Read the model definition and answer for the solid it produces. Units are mm, in the model's axes. A direction names the side the tool comes from. Round coordinates to 2 decimals unless told otherwise and drop trailing zeros. Order: outer loops, then holes, each group sorted by start corner. A loop starts at its lowest first (then second) coordinate and runs counter-clockwise, first axis right, second up. Notation, with made-up numbers: M 51.25,-30.5 L 81.25,-30.5 A18 cw 81.25,-9.5 Z; hole C -17,-3 d7. An arc over 180 degrees is marked long. Answer as CSV lines item,"result".
```python
from build123d import *

# Parameters (mm, degrees)
BOSS_EXTRUDE1_DEPTH = 9
CUT_EXTRUDE1_DEPTH  = 1.5


with BuildPart() as part:
    # Sketch1 → Boss-Extrude1 (new, symmetric)
    with BuildSketch(Plane.XY):
        with BuildLine():
            Line((-0.064848747, 6.937253933), (-8.564848747, 6.937253933))
            Line((-8.564848747, 6.937253933), (-8.564848747, 7.937253933))
            Line((-8.564848747, 7.937253933), (0, 7.937253933))
            ThreePointArc((0, 7.937253933), (5, 5.291502622), (7, 0))
            ThreePointArc((7, 0), (6.838022738, -1.497145631), (6.359587132, -2.925004532))
            Line((6.359587132, -2.925004532), (5.451074684, -2.507146742))
            ThreePointArc((5.451074684, -2.507146742), (5.861162347, -1.283267683), (6, 0))
            ThreePointArc((6, 0), (4.270012276, 4.607273664), (-0.064848747, 6.937253933))
        make_face()
    extrude(amount=BOSS_EXTRUDE1_DEPTH, both=True)

    # Sketch2 → Cut-Extrude1 (cut)
    with BuildSketch(Plane.XY.offset(9)):
        with BuildLine():
            Line((5.451074684, -2.507146742), (6.359587132, -2.925004532))
            ThreePointArc((6.359587132, -2.925004532), (6.838022738, -1.497145631), (7, 0))
            ThreePointArc((7, 0), (5.923664522, 4.007850993), (2.984282604, 6.937253933))
            Line((2.984282604, 6.937253933), (-0.064848747, 6.937253933))
            ThreePointArc((-0.064848747, 6.937253933), (4.270012276, 4.607273664), (6, 0))
            ThreePointArc((6, 0), (5.861162347, -1.283267683), (5.451074684, -2.507146742))
        make_face()
    cut_extrude1 = extrude(amount=-CUT_EXTRUDE1_DEPTH, mode=Mode.SUBTRACT)

    # Mirror1: Cut-Extrude1 across plane
    add(cut_extrude1.mirror(Plane.XY), mode=Mode.SUBTRACT)


solid = part.part
```
Item 1: A tool of negligible diameter and unlimited length cuts with its end or side. For faces 4 (the face through (-2.7, 7.4, -9)), 5 (the face through (4.32, 4.55, 0.11)), 6 (the face through (6, 3, -7.5)), 7 (the face through (6, 3, 7.5)), from which of +Z, -Z, +X, -X, +Y, -Y can it reach the whole face along a straight path? Write none if from no direction.
Ans:
face 4,"-Z, +X, -X, +Y, -Y"
face 5,"+Z, -Z, -X"
face 6,"-Z, +X, -X, -Y"
face 7,"+Z, +X, -X, -Y"
Item 2: Find the intervals of material crossed by probe 1 along Y at (x, z) = (-6.75, -7.5); probe 2 along X at (y, z) = (3.75, -5); probe 3 along X at (y, z) = (5.5, 2.5), in increasing order. Write a range as [from, to].
Ans:
probe 1,"[6.94, 7.94]"
probe 2,"[4.91, 6.07]"
probe 3,"[3.33, 4.81]"
Item 3: Determine the mould class of faces 1 (the face through (4.9, 5.4, 0.1)), 2 (the face through (-4, 6.937, 0)), 3 (the face through (5.857, -1.301, 0.105)) for opening direction Y: +Y half, -Y half, draft (parallel to the pull), parting line (faces both ways), or undercut.
Ans:
face 1,"+Y half"
face 2,"-Y half"
face 3,"undercut"
Item 4: A cutting plane is placed at B-B, the plane x = 1.25. Determine the outline of the cut face in (y, z).
Ans:
outline,"M 6.63,-7.5 L 6.94,-7.5 L 6.94,-9 L 7.68,-9 L 7.68,9 L 6.94,9 L 6.94,7.5 L 6.63,7.5 Z"
Item 5: A cutting plane is placed at C-C, the plane y = -1.25. Determine the outline of the cut face in (x, z).
Ans:
outline,"M 5.87,-7.5 L 6.89,-7.5 L 6.89,7.5 L 5.87,7.5 Z"
Item 6: A cutting plane is placed at D-D, the plane x = -7.5. Determine the outline of the cut face in (y, z), and give its area (3 significant figures).
Ans:
outline,"M 6.94,-9 L 7.94,-9 L 7.94,9 L 6.94,9 Z"
area,"18.0 mm2"
Item 7: Flat-ended cylindrical pins translate along their axes: pin 1 (6 mm diameter, centred on y = 2, z = 5, fed in from -X); pin 2 (9 mm diameter, centred on x = -3.5, z = 2.5, fed in from -Y); pin 3 (1 mm diameter, centred on x = 3.5, z = -2.5, fed in from +Y); pin 4 (2 mm diameter, centred on x = 3.5, y = 3.5, fed in from +Z). Find the tip coordinate at first contact, or state that the pin passes through.
Ans:
pin 1,"x = 3.9"
pin 2,"y = 6.71"
pin 3,"y = 6.93"
pin 4,"through"
Item 8: A cutting plane is placed at A-A, the plane z = 1.25. Determine the outline of the cut face in (x, y) (3 decimals).
Ans:
outline,"M -8.565,6.937 L -0.065,6.937 A7 cw 6,0 A6 cw 5.451,-2.507 L 6.36,-2.925 A7 ccw 7,0 A8 ccw 0,7.937 L -8.565,7.937 Z"
